Design review of the part built by this model. Coordinates are the model's own, in mm. A direction names the side the tool comes from. Give positions to 0.01 mm unless a question says otherwise; leave off trailing zeros. Loops run counter-clockwise (first coordinate to the right, second up) from the corner with the lowest first, then second, coordinate; pieces in that order, holes last. Notation, with made-up numbers: (-36.5, 85.5) -> (-26.5, 85.5) arc R26 cw to (-26.5, 106.5) -> close; hole circle Ø7 at (28.25, 80). An arc over 180 degrees is marked (long way). Answer as CSV lines item,"result".
from build123d import *

# Parameters (mm, degrees)
SKETCH1_W           = 95
SKETCH1_H           = 95
SKETCH1_R           = 37.5
BOSS_EXTRUDE1_DEPTH = 2
SKETCH3_W           = 12
SKETCH3_H           = 4
SKETCH3_W_2         = 11
CUT_EXTRUDE5_DEPTH  = 68.294130502
FILLET1_R           = 5


with BuildPart() as part:
    # Sketch1 → Boss-Extrude1 (new, symmetric)
    with BuildSketch(Plane(origin=(0, 0, 0), x_dir=(1, 0, 0), z_dir=(0, 1, 0))):
        Rectangle(SKETCH1_W, SKETCH1_H)
        with Locations(Location((0, 0, 0), (0, 0, 270))):
            Circle(SKETCH1_R, mode=Mode.SUBTRACT)
    extrude(amount=BOSS_EXTRUDE1_DEPTH, both=True)

    # Sketch3 → Cut-Extrude5 (cut, through all)
    with BuildSketch(Plane(origin=(0, 2, 0), x_dir=(1, 0, 0), z_dir=(0, 1, 0))):
        with Locations((-41.5, 37.5)):
            Rectangle(SKETCH3_W, SKETCH3_H)
        with Locations((-22, 37.5)):
            Rectangle(SKETCH3_W_2, SKETCH3_H)
        with Locations((22, 37.5)):
            Rectangle(SKETCH3_W_2, SKETCH3_H)
        with Locations((41.5, 37.5)):
            Rectangle(SKETCH3_W, SKETCH3_H)
        with Locations((41.5, -37.5)):
            Rectangle(SKETCH3_W, SKETCH3_H)
        with Locations((22, -37.5)):
            Rectangle(SKETCH3_W_2, SKETCH3_H)
        with Locations((-22, -37.5)):
            Rectangle(SKETCH3_W_2, SKETCH3_H)
        with Locations((-41.5, -37.5)):
            Rectangle(SKETCH3_W, SKETCH3_H)
    extrude(amount=-CUT_EXTRUDE5_DEPTH, mode=Mode.SUBTRACT)

    # Fillet1
    fillet1_edges = [part.edges().sort_by_distance(p)[0] for p in [
        (47.5, 0, 47.5),
        (47.5, 0, -47.5),
    ]]
    fillet(fillet1_edges, radius=FILLET1_R)


solid = part.part
Q1. Clearance check with flat-ended pins moving along their axes: pin 1 Ø1.2 at (y, z) = (0, -37) entering from -X; pin 2 Ø1.5 at (x, z) = (-23, -28) entering from +Y. State where each tip first meets the part, or that it passes through.
Filled sheet:
pin 1,"stops at x = -35.5"
pin 2,"passes through"
Q2. We need section A-A, the plane z = 0. State the section outline as (x, y) points.
Filled sheet:
outline,"(-47.5, -2) -> (-37.5, -2) -> (-37.5, 2) -> (-47.5, 2) -> close; (37.5, -2) -> (47.5, -2) -> (47.5, 2) -> (37.5, 2) -> close"
Q3. To check wall thickness, follow probe 1 along Z at (x, y) = (38.5, 1.4); probe 2 along X at (y, z) = (0.45, 39); probe 3 along Z at (x, y) = (-1, -0.8). State the ranges of each line that lie inside material, in increasing order. Write a range as from..to.
Filled sheet:
probe 1,"z = -47.5..-39.5, -35.5..35.5, 39.5..47.5"
probe 2,"x = -35.5..-27.5, -16.5..16.5, 27.5..35.5"
probe 3,"z = -47.5..-37.49, 37.49..47.5"
Q4. The part is to be moulded in two halves that separate along X. For faces 4 (the cylindrical face through (46, 0.03, 46.07)), 5 (the flat face through (-35.5, 0, -37)), 6 (the flat face through (22, 0, -39.5)), say which applies: pulls with the +X half, pulls with the -X half, needs draft (parallel to the pull), parting line crosses it, or undercut.
Filled sheet:
face 4,"pulls with the +X half"
face 5,"pulls with the -X half"
face 6,"undercut"
Q5. We need section C-C, the plane y = -0.35. State how many separate pieces and enclosed holes the cut face has, and give its area (3 significant figures).
Filled sheet:
separate pieces,"1"
enclosed holes,"5"
area,"4,230 mm^2"
Q6. We need section B-B, the plane x = 13.5. State the section outline as (y, z) points.
Filled sheet:
outline,"(-2, -47.5) -> (2, -47.5) -> (2, -34.99) -> (-2, -34.99) -> close; (-2, 34.99) -> (2, 34.99) -> (2, 47.5) -> (-2, 47.5) -> close"
Q7. For faces 1 (the flat face through (-47.5, 0, 0)), 2 (the flat face through (35.5, 0, -37)), 3 (the flat face through (16.5, 0, -37)), list the 3-axis set-ups (+Z, -Z, +X, -X, +Y, -Y) from which the entire face can be reached by the end or side of a thin tool; tool diameter is ignored.
Filled sheet:
face 1,"+Z, -Z, -X, +Y, -Y"
face 2,"+X, +Y, -Y"
face 3,"+Y, -Y"
